For this review, take the finished solid that the model builds, in its own axes (mm). A direction names the side the tool comes from. Give positions to 0.01 mm unless a question says otherwise; leave off trailing zeros. Write each loop counter-clockwise with the first axis right and the second up, starting at its lowest first coordinate (ties: lowest second). Pieces come first, ordered by that corner, then holes. Notation, with made-up numbers: (62.5, 27) -> (121.5, 27) arc R21 cw to (121.5, 58) -> close; hole circle Ø11 at (9.5, 67). An arc over 180 degrees is marked (long way). Write item = value, one per line.
```python
from build123d import *

# Parameters (mm, degrees)
SKETCH1_W           = 25.4
SKETCH1_H           = 12.7
BOSS_EXTRUDE1_DEPTH = 3.175
SKETCH2_W           = 6.4262
SKETCH2_H           = 3.175
BOSS_EXTRUDE2_DEPTH = 3.175
CUT_EXTRUDE1_DEPTH  = 3.175
SKETCH4_R           = 3.175
CUT_EXTRUDE2_DEPTH  = 4.175


with BuildPart() as part:
    # Sketch1 → Boss-Extrude1 (new body)
    with BuildSketch(Plane(origin=(0, 0, 0), x_dir=(1, 0, 0), z_dir=(0, 1, 0))):
        Rectangle(SKETCH1_W, SKETCH1_H)
    extrude(amount=BOSS_EXTRUDE1_DEPTH)

    # Sketch2 → Boss-Extrude2 (add)
    with BuildSketch(Plane.XY.offset(6.35)):
        with Locations((9.4869, 1.5875)):
            Rectangle(SKETCH2_W, SKETCH2_H)
        with Locations((-3.2893, 1.5875)):
            Rectangle(SKETCH2_W, SKETCH2_H)
    boss_extrude2 = extrude(amount=BOSS_EXTRUDE2_DEPTH)

    # Mirror1: Boss-Extrude2 across plane
    add(boss_extrude2.mirror(Plane.XY))

    # Sketch3 → Cut-Extrude1 (cut)
    with BuildSketch(Plane(origin=(0, 3.175, 0), x_dir=(1, 0, 0), z_dir=(0, 1, 0))):
        Polygon((-6.5024, -6.35), (-12.7, 6.35), (-12.7, -6.35), align=None)
    extrude(amount=-CUT_EXTRUDE1_DEPTH, mode=Mode.SUBTRACT)

    # Sketch4 → Cut-Extrude2 (cut, through all)
    with BuildSketch(Plane(origin=(0, 3.175, 0), x_dir=(1, 0, 0), z_dir=(0, 1, 0))):
        with Locations((-2.505931508, 0)):
            Circle(SKETCH4_R)
        with Locations((6.741308704, 0)):
            Circle(SKETCH4_R)
    extrude(amount=-CUT_EXTRUDE2_DEPTH, mode=Mode.SUBTRACT)


solid = part.part
```
(1) To check wall thickness, follow probe 1 along X at (y, z) = (1.8, 0); probe 2 along X at (y, z) = (2.4, -2); probe 3 along Z at (x, y) = (8.75, 2.7) (3 decimals). State the ranges of each line that lie inside material, in increasing order.
Answers below:
probe_1 = -9.6 to -5.68, 0.67 to 3.57, 9.92 to 12.7
probe_2 = -10.58 to -4.97, -0.04 to 4.28, 9.21 to 12.7
probe_3 = -9.525 to -2.459, 2.459 to 9.525
(2) Take a section at C-C (z = 0). Write out the cut boundary in (x, y) (3 decimals), plus the area to 3 significant figures.
Answers below:
outline = (-9.601, 0) -> (-5.681, 0) -> (-5.681, 3.175) -> (-9.601, 3.175) -> close; (0.669, 0) -> (3.566, 0) -> (3.566, 3.175) -> (0.669, 3.175) -> close; (9.916, 0) -> (12.7, 0) -> (12.7, 3.175) -> (9.916, 3.175) -> close
area = 30.5 mm^2
(3) The part is to be moulded in two halves that separate along X. For faces 5 (the face through (9.674, 1.61, 1.216)), 6 (the face through (-9.558, 1.61, 0.089)), 7 (the face through (-10, 2, -6.35)), 8 (the face through (-3.2, 1.6, 3.1)), say which applies: released by +X, released by -X, zero draft, split by the parting line, or undercut.
Answers below:
face_5 = undercut
face_6 = released by -X
face_7 = zero draft
face_8 = undercut
(4) Take a section at B-B (x = 4.5). Write out the cut boundary in (y, z) (3 decimals).
Answers below:
outline = (0, -6.35) -> (3.175, -6.35) -> (3.175, -2.249) -> (0, -2.249) -> close; (0, 2.249) -> (3.175, 2.249) -> (3.175, 6.35) -> (0, 6.35) -> close
(5) Take a section at A-A (y = 1.9). Write out the cut boundary in (x, z) (3 decimals).
Answers below:
outline = (-12.7, -6.35) -> (-6.502, -6.35) -> (-6.502, -9.525) -> (-0.076, -9.525) -> (-0.076, -6.35) -> (6.274, -6.35) -> (6.274, -9.525) -> (12.7, -9.525) -> (12.7, 9.525) -> (6.274, 9.525) -> (6.274, 6.35) -> (-0.076, 6.35) -> (-0.076, 9.525) -> (-6.502, 9.525) -> (-6.502, 6.35) -> close; hole circle Ø6.35 at (-2.506, 0); hole circle Ø6.35 at (6.741, 0)
(6) Tool access review of faces 1 (the face through (3, 3.175, 0)), 2 (the face through (6.274, 2, 8)), 3 (the face through (-6.502, 2, 8)), 4 (the face through (6.274, 2, -8)): name each direction out of +Z, -Z, +X, -X, +Y, -Y from which nothing blocks a thin tool from reaching the whole face with its end or side.
Answers below:
face_1 = +Z, -Z, +X, -X, +Y
face_2 = +Z, +Y, -Y
face_3 = +Z, -X, +Y, -Y
face_4 = -Z, +Y, -Y
(7) For pin 1 (1.5 mm diameter, centred on y = 2.5, z = 2, fed in from -X); pin 2 (1.6 mm diameter, centred on y = 2, z = 8, fed in from -X); pin 3 (1.6 mm diameter, centred on x = 4.5, y = 1.5, fed in from +Z), all flat-tipped, find the tip position at first contact; note any pin that passes through.
Answers below:
pin_1 = -8.99
pin_2 = -6.5
pin_3 = 6.35
(8) Take a section at D-D (x = -3). Write out the cut boundary in (y, z) (3 decimals), plus the area to 3 significant figures.
Answers below:
outline = (0, -9.525) -> (3.175, -9.525) -> (3.175, -3.136) -> (0, -3.136) -> close; (0, 3.136) -> (3.175, 3.136) -> (3.175, 9.525) -> (0, 9.525) -> close
area = 40.6 mm^2
